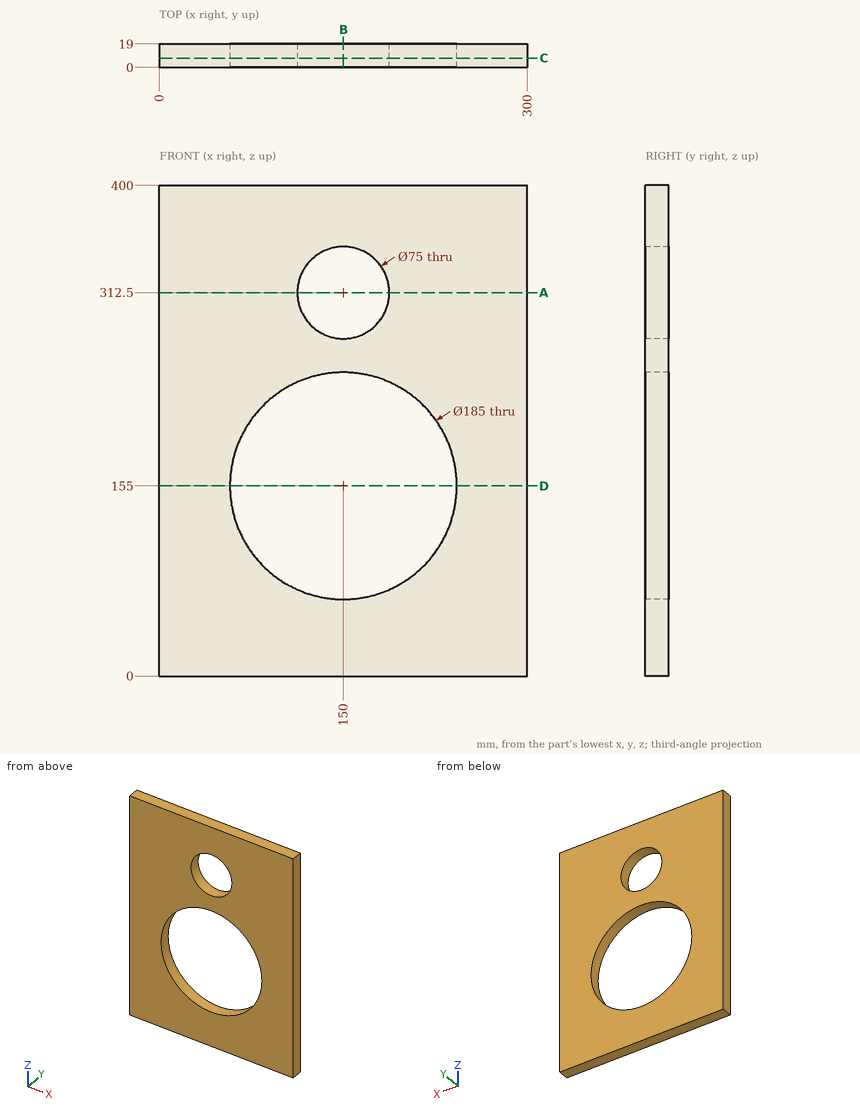
Source: three-view drawing plus pictorial views. Frame: mm from the lowest corner of the part. Give positions to 0.01 mm unless a question says otherwise; leave off trailing zeros. Order: outer loops, then holes, each group sorted by start corner. A loop starts at its lowest first (then second) coordinate and runs counter-clockwise, first axis right, second up. Notation, with made-up numbers: (-17, 33) - (33, 33) arc R19 ccw to (33, 50) - close; hole circle Ø1 at (82, -27.5). An arc over 180 degrees is marked (long way). Put each result on its own line as item: value.
Item 1: Section query B-B, the plane x = 150. Return loops of the section in (y, z).
Found:
outline: (0, 0) - (19, 0) - (19, 62.5) - (0, 62.5) - close; (0, 247.5) - (19, 247.5) - (19, 275) - (0, 275) - close; (0, 350) - (19, 350) - (19, 400) - (0, 400) - close
Item 2: Ray query, L1, parallel to Z at x = 150, y = 11.25; L2, parallel to Z at x = 129, y = 1.25; L3, parallel to X at y = 11.5, z = 149. Return the intervals inside material, ascending. Write a range as from..to.
Found:
L1: z = 0..62.5, 247.5..275, 350..400
L2: z = 0..64.92, 245.08..281.43, 343.57..400
L3: x = 0..57.69, 242.31..300
Item 3: Section query C-C, the plane y = 7.5. Return loops of the section in (x, z), then the cut area to 3 significant figures.
Found:
outline: (0, 0) - (300, 0) - (300, 400) - (0, 400) - close; hole circle Ø185 at (150, 155); hole circle Ø75 at (150, 312.5)
area: 88,700 mm^2
Item 4: Section query A-A, the plane z = 312.5. Return loops of the section in (x, y).
Found:
outline: (0, 0) - (112.5, 0) - (112.5, 19) - (0, 19) - close; (187.5, 0) - (300, 0) - (300, 19) - (187.5, 19) - close
Item 5: Section query D-D, the plane z = 155. Return loops of the section in (x, y), then the cut area to 4 significant figures.
Found:
outline: (0, 0) - (57.5, 0) - (57.5, 19) - (0, 19) - close; (242.5, 0) - (300, 0) - (300, 19) - (242.5, 19) - close
area: 2,185 mm^2
